```python
from build123d import *

# Parameters (mm, degrees)
SKETCH1_R      = 1.5875
EXTRUDE1_DEPTH = 1.27


with BuildPart() as part:
    # Sketch1 → Extrude1 (new body)
    with BuildSketch(Plane.XY):
        with BuildLine():
            Line((0, 15.8496), (-0.0254, 15.875))
            Line((-0.0254, 15.875), (-64.77, 15.875))
            ThreePointArc((-64.77, 15.875), (-67.464076836, 14.759076836), (-68.58, 12.065))
            Line((-68.58, 12.065), (-68.58, 3.81))
            ThreePointArc((-68.58, 3.81), (-67.464076836, 1.115923164), (-64.77, 0))
            Line((-64.77, 0), (-0.0254, 0))
            Line((-0.0254, 0), (0, 0.0254))
            Line((0, 0.0254), (0, 15.8496))
        make_face()
        with Locations((-62.23, 7.9375)):
            Circle(SKETCH1_R, mode=Mode.SUBTRACT)
    extrude(amount=EXTRUDE1_DEPTH)


solid = part.part
```
Could you check a few things on this model? Use its own coordinates, in mm. Round coordinates to 2 decimals unless told otherwise and drop trailing zeros. Loops run counter-clockwise (first coordinate to the right, second up) from the corner with the lowest first, then second, coordinate; pieces in that order, holes last. Notation, with made-up numbers: M 37.5,59 L 58.5,59 A24 cw 58.5,86 Z; hole C 82.25,86.5 d7. An arc over 180 degrees is marked long. Write item = value, one per line.
1. Thinking about a two-plate mould opening in Y: for faces 1 (the face through (-35, 8, 1.27)), 2 (the face through (-67.494, 1.146, 0.626)), 3 (the face through (-63.816, 8.007, 0.626)), which applies, +Y half, -Y half, draft (parallel to the pull), parting line (faces both ways), or undercut?
Results below:
face_1 = draft
face_2 = -Y half
face_3 = undercut
2. I want a section at A-A, the plane x = -62.23. Write out the boundary of the cut face in (y, z) (3 decimals).
Results below:
outline = M 0,0 L 6.35,0 L 6.35,1.27 L 0,1.27 Z; M 9.525,0 L 15.875,0 L 15.875,1.27 L 9.525,1.27 Z
3. I want a section at B-B, the plane y = 7.25. Write out the boundary of the cut face in (x, z).
Results below:
outline = M -68.58,0 L -63.66,0 L -63.66,1.27 L -68.58,1.27 Z; M -60.8,0 L 0,0 L 0,1.27 L -60.8,1.27 Z
4. I need wall thicknesses on probe 1 along Y at (x, z) = (-62.23, 0.4) (3 decimals); probe 2 along X at (y, z) = (8, 0.2); probe 3 along X at (y, z) = (7.75, 1.2). Which ranges of each line are inside material? Lowest first, please.
Results below:
probe_1 = 0 to 6.35, 9.525 to 15.875
probe_2 = -68.58 to -63.82, -60.64 to 0
probe_3 = -68.58 to -63.81, -60.65 to 0
